Source: CAD feature listing. Evaluate the final solid. Frame: model axes, mm. A direction names the side the tool comes from. Coordinates: 2 decimals unless noted, no trailing zeros. Write each loop counter-clockwise with the first axis right and the second up, starting at its lowest first coordinate (ties: lowest second). Pieces come first, ordered by that corner, then holes. Notation, with made-up numbers: (31, -16.75) - (79, -16.75) arc R22 ccw to (79, 7.25) - close; hole circle Ø2 at (10.25, -31.75). An arc over 180 degrees is marked (long way). One line per question, with ' | ' between items.
from build123d import *

# Parameters (mm, degrees)
HOLE_WIZARD_M61_D        = 5
HOLE_WIZARD_M61_DEPTH    = 18
HOLE_WIZARD_M61_TIP      = 1.502151548
CHAMFER_2_SIZE           = 1
SKETCH_12_R              = 18
SKETCH_12_R_2            = 15
CUT_EXTRUDE_1_DEPTH      = 4
SKETCH_11_W              = 65
SKETCH_11_H              = 10
PATTERN_CIRCULAR_1_COUNT = 6
CHAMFER_3_SIZE           = 5
CHAMFER_4_SIZE           = 2
CHAMFER_5_SIZE           = 1


with BuildPart() as part:
    # Эскиз1 → Повернуть1 (revolve)
    with BuildSketch(Plane.XY, mode=Mode.PRIVATE) as revolve_1_sk:
        Polygon((-48, 15), (-48, 30), (-40, 30), (-40, 47.5), (40, 47.5), (40, 32.5), (18, 32.5), (18, 23.5), (-18, 23.5), (-18, 21), (-21, 21), (-21, 15), align=None)
    revolve(revolve_1_sk.sketch.rotate(Axis((0, 0, 0), (1, 0, 0)), 90), axis=Axis((0, 0, 0), (1, 0, 0)))

    # Отверстие обработанное метчиком M61
    with Locations(Plane.ZY.offset(48)):
        with Locations((0, 24), (20.784609691, 12), (20.784609691, -12), (0, -24), (-20.784609691, -12), (-20.784609691, 12)):
            Hole(HOLE_WIZARD_M61_D / 2, depth=HOLE_WIZARD_M61_DEPTH)
            with Locations((0, 0, -(HOLE_WIZARD_M61_DEPTH + HOLE_WIZARD_M61_TIP / 2))):  # 118° drill point
                Cone(0, HOLE_WIZARD_M61_D / 2, HOLE_WIZARD_M61_TIP, mode=Mode.SUBTRACT)

    # Эскиз10 → Отверстие обработанное метчиком M44 (revolve, cut)
    with BuildSketch(Plane(origin=(18, 27.5, 0), x_dir=(0, 0, -1), z_dir=(0, 1, 0))):
        Polygon((0, 0), (0, 16.991420021), (1.65, 16), (1.65, 0.85), (2.5, 0), align=None)
    hole_wizard_m44 = revolve(axis=Axis((24.35, 27.5, 0), (-1, 0, 0)), mode=Mode.SUBTRACT)

    # Фаска2
    chamfer_2_edges = [part.edges().sort_by_distance(p)[0] for p in [
        (-48, 12, -18.284609691),
        (-48, -12, -18.284609691),
        (-48, -24, 2.5),
        (-48, -12, 23.284609691),
        (-48, 12, 23.284609691),
        (-48, 24, 2.5),
    ]]
    chamfer(chamfer_2_edges, length=CHAMFER_2_SIZE)

    # Эскиз12 → Вырез-Вытянуть1 (cut)
    with BuildSketch(Plane.ZY.offset(48)):
        Circle(SKETCH_12_R)
        Circle(SKETCH_12_R_2, mode=Mode.SUBTRACT)
    extrude(amount=-CUT_EXTRUDE_1_DEPTH, mode=Mode.SUBTRACT)

    # Эскиз11 → Вырез-Повернуть1 (revolve, cut)
    with BuildSketch(Plane.XY, mode=Mode.PRIVATE) as cut_revolve_1_sk:
        with Locations((-7.5, 42.5)):
            Rectangle(SKETCH_11_W, SKETCH_11_H)
    revolve(cut_revolve_1_sk.sketch.rotate(Axis((0, 0, 0), (-1, 0, 0)), 270), axis=Axis((0, 0, 0), (-1, 0, 0)), mode=Mode.SUBTRACT)

    # Круговой массив1: Отверстие обработанное метчиком M44 ×6 about axis
    pattern_circular_1_axis = Axis((0, 0, 0), (1, 0, 0))
    for i in range(1, PATTERN_CIRCULAR_1_COUNT):
        add(hole_wizard_m44.rotate(pattern_circular_1_axis, i * 360 / PATTERN_CIRCULAR_1_COUNT), mode=Mode.SUBTRACT)

    # Фаска3
    chamfer_3_edges = [part.edges().sort_by_distance(p)[0] for p in [
        (25, 0, -37.5),
    ]]
    chamfer(chamfer_3_edges, length=CHAMFER_3_SIZE)

    # Фаска4
    chamfer_4_edges = [part.edges().sort_by_distance(p)[0] for p in [
        (40, 0, -32.5),
    ]]
    chamfer(chamfer_4_edges, length=CHAMFER_4_SIZE)

    # Фаска5
    chamfer_5_edges = [part.edges().sort_by_distance(p)[0] for p in [
        (18, 0, -23.5),
        (-44, 0, -15),
        (-48, 0, -18),
        (-40, 0, -37.5),
        (-48, 0, -30),
    ]]
    chamfer(chamfer_5_edges, length=CHAMFER_5_SIZE)


solid = part.part
Item 1: Ray query, line 1 along Y through (x, z) = (-38, 0); line 2 along Y through (x, z) = (-36, -0.5); line 3 along Y through (x, z) = (2.5, 21.5). Return the intervals inside material, ascending. Write a range as [from, to].
Check sheet entries:
line 1: [-37.5, -26.5], [-21.5, -15], [15, 21.5], [26.5, 37.5] | line 2: [-37.5, -26.45], [-21.55, -14.99], [14.99, 21.55], [26.45, 37.5] | line 3: [-30.72, -9.49], [9.49, 30.72]
Item 2: Cut plane A-A on x = -1. Return loops of the section in (y, z), and give its area (3 significant figures).
Check sheet entries:
outline: circle Ø75 at (0, 0); hole circle Ø47 at (0, 0) | area: 2,680 mm²
Item 3: Pin query (flat end, axial travel): pin 1 Ø5.5 at (y, z) = (27.5, 0) entering from +X; pin 2 Ø6 at (y, z) = (-12, 20.78) entering from -X; pin 3 Ø2 at (x, z) = (7.5, -24.5) entering from +Y. Return the tip coordinate at first contact, or that it passes through.
Check sheet entries:
pin 1: x = 18 | pin 2: x = -47.5 | pin 3: y = 29.22
Item 4: Mould query, pull axis Z, two halves, no side actions, for faces 1 (the face through (40, -25, 24)), 2 (the face through (9.681, -25.864, -0.215)), 3 (the face through (20.313, 11.358, 36.067)). Classes: pulls with the +Z half, pulls with the -Z half, needs draft (parallel to the pull), parting line crosses it, or undercut.
Check sheet entries:
face 1: needs draft | face 2: undercut | face 3: parting line crosses it
Item 5: Access query for faces 4 (the face through (-38.38, -13.52, -18.8)), 5 (the face through (9.68, -13.12, -25.34)). Directions: +Z, -Z, +X, -X, +Y, -Y. A direction counts if a zero-diameter tool reaches every point of the face in a straight line with its end or side. Return the directions, or none.
Check sheet entries:
face 4: -X | face 5: +X
